```python
from build123d import *

# Parameters (mm, degrees)
F0_W     = 50.8
F0_H     = 111.125
F1_DEPTH = 15.875
F3_D     = 6.9088
F3_DEPTH = 11.938
F3_TIP   = 2.0756129224


with BuildPart() as f1:
    # F0 (on Front) → F1 (new body, symmetric)
    with BuildSketch(Plane.XZ):
        Rectangle(F0_W, F0_H)
    extrude(amount=F1_DEPTH, both=True)

    # F3
    with Locations(Plane.XZ.offset(15.875)):
        with Locations((-11.1125, 45.9105), (11.1125, 45.9105), (-11.1125, 20.5105), (11.1125, 20.5105)):
            Hole(F3_D / 2, depth=F3_DEPTH)
            with Locations((0, 0, -(F3_DEPTH + F3_TIP / 2))):  # 118° drill point
                Cone(0, F3_D / 2, F3_TIP, mode=Mode.SUBTRACT)


solid = f1.part
```
Check sheet for the modelled part. Datum: model origin and axes. Units: mm. A direction names the side the tool comes from. Give positions to 0.01 mm unless a question says otherwise; leave off trailing zeros. Order: outer loops, then holes, each group sorted by start corner. A loop starts at its lowest first (then second) coordinate and runs counter-clockwise, first axis right, second up. Notation, with made-up numbers: M 60,14.5 L 104,14.5 A37 cw 104,52.5 Z; hole C 7,65 d10. An arc over 180 degrees is marked long. Answer in a Markdown table with one row per item. Add a question column.
Q1. Access from +Z, -Z, +X, -X, +Y, -Y to the whole of each face (thin tool, end or side, straight path). Record for faces 1 (the flat face through (0, 15.875, 1)), 2 (the cylindrical face through (-10.36, -9.82, 42.54)).
Q2. Release check for a two-part mould opening along X. For faces 3 (the flat face through (0, 0, 55.562)), 4 (the conical face through (-10.84, -2.22, 19.98)), 5 (the flat face through (-25.4, 0, -1)) record: released by +X, released by -X, zero draft, split by the parting line, or undercut.
Q3. Thickness scan on L1, parallel to Z at x = -11, y = -7; L2, parallel to Z at x = 8, y = -5.5; L3, parallel to X at y = -7, z = 21.5. Record the ranges inside material, lowest first.
Q4. Sectioned sample at A-A, the plane y = -9. Record the boundary of the cut face in (x, z).
Verdict:
| question | item | result |
|---|---|---|
| 1 | face 1 | +Z, -Z, +X, -X, +Y |
| 1 | face 2 | -Y |
| 2 | face 3 | zero draft |
| 2 | face 4 | undercut |
| 2 | face 5 | released by -X |
| 3 | L1 | -55.56 to 17.06, 23.96 to 42.46, 49.36 to 55.56 |
| 3 | L2 | -55.56 to 19.01, 22.01 to 44.41, 47.41 to 55.56 |
| 3 | L3 | -25.4 to -14.42, -7.8 to 7.8, 14.42 to 25.4 |
| 4 | outline | M -25.4,-55.56 L 25.4,-55.56 L 25.4,55.56 L -25.4,55.56 Z; hole C -11.11,20.51 d6.91; hole C -11.11,45.91 d6.91; hole C 11.11,20.51 d6.91; hole C 11.11,45.91 d6.91 |
